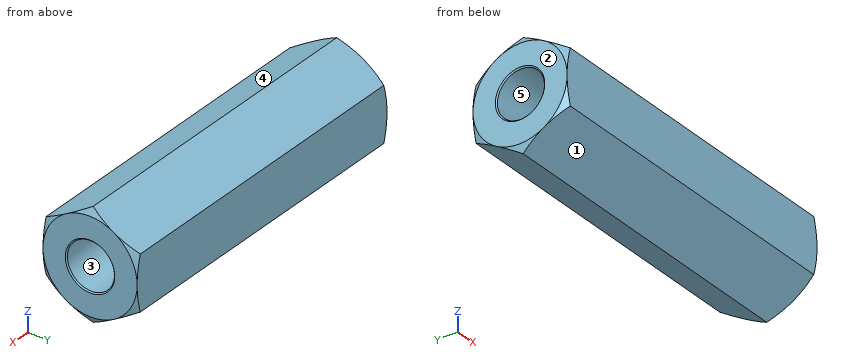
from build123d import *

# Parameters (mm, degrees)
BOSS_EXTRUDE1_DEPTH = 28
SKETCH4_OUTSIDE_W   = 117.808
SKETCH4_OUTSIDE_H   = 116.57
SKETCH4_OUTSIDE_R   = 4
CUT_EXTRUDE1_DEPTH  = 29
CUT_EXTRUDE1_TAPER  = 60
SKETCH5_OUTSIDE_W   = 117.808
SKETCH5_OUTSIDE_H   = 116.57
SKETCH5_OUTSIDE_R   = 4
CUT_EXTRUDE2_DEPTH  = 29
CUT_EXTRUDE2_TAPER  = 60


with BuildPart() as part:
    # Sketch2 → Boss-Extrude1 (new body)
    with BuildSketch(Plane(origin=(0, 0, 0), x_dir=(0, 0, -1), z_dir=(1, 0, 0))):
        Polygon((2.309401077, 4), (-2.309401077, 4), (-4.618802154, 0), (-2.309401077, -4), (2.309401077, -4), (4.618802154, 0), align=None)
    extrude(amount=BOSS_EXTRUDE1_DEPTH)

    # Sketch3 → Cut-Revolve1 (revolve, cut)
    with BuildSketch(Plane.XY):
        Polygon((0, 2.1), (0.1, 2), (11.1, 2), (11.1, 0), (0, 0), align=None)
        Polygon((28, 0), (16.9, 0), (16.9, 2), (27.9, 2), (28, 2.1), align=None)
    revolve(axis=Axis((0, 0, 0), (1, 0, 0)), mode=Mode.SUBTRACT)

    # Sketch4 outside → Cut-Extrude1 (cut, through all)
    with BuildSketch(Plane.ZY):
        Rectangle(SKETCH4_OUTSIDE_W, SKETCH4_OUTSIDE_H)
        Circle(SKETCH4_OUTSIDE_R, mode=Mode.SUBTRACT)
    extrude(amount=-CUT_EXTRUDE1_DEPTH, taper=CUT_EXTRUDE1_TAPER, mode=Mode.SUBTRACT)

    # Sketch5 outside → Cut-Extrude2 (cut, through all)
    with BuildSketch(Plane(origin=(28, 0, 0), x_dir=(0, 0, -1), z_dir=(1, 0, 0))):
        Rectangle(SKETCH5_OUTSIDE_W, SKETCH5_OUTSIDE_H)
        Circle(SKETCH5_OUTSIDE_R, mode=Mode.SUBTRACT)
    extrude(amount=-CUT_EXTRUDE2_DEPTH, taper=CUT_EXTRUDE2_TAPER, mode=Mode.SUBTRACT)


solid = part.part
CAD build for the part. Positions are in the model's coordinates, mm. Face numbers are marked on the shaded views. A direction names the side the tool comes from. Coordinates: 2 decimals unless noted, no trailing zeros. Loops run counter-clockwise (first coordinate to the right, second up) from the corner with the lowest first, then second, coordinate; pieces in that order, holes last. Notation, with made-up numbers: (0.25, -12) - (12.25, -12) arc R24 ccw to (12.25, 2) - close; hole circle Ø9 at (2.5, -40). An arc over 180 degrees is marked (long way). Write item = value, one per line. Start each with the question number.
Q1. Pull direction Z, two halves, no side cores. Call the marked faces 1, 2 and 3: pulls with the +Z half, pulls with the -Z half, needs draft (parallel to the pull), parting line crosses it, or undercut.
Q2. Cut at A-A, the plane x = 9.75. List the corners of the cut face in (y, z).
Q3. Flat gauge pins, fed straight in: pin 1 Ø3 at (y, z) = (0, 0) entering from +X; pin 2 Ø1 at (x, y) = (23.5, -2) entering from +Z; pin 3 Ø2 at (x, y) = (7.5, -1.5) entering from +Z. Where does each tip first touch, or does it go through?
Q4. Drill centre lines: L1, parallel to X at y = -1, z = -1; L2, parallel to Z at x = 5.25, y = 0.75; L3, parallel to Y at x = 9.5, z = -1. Where is each one in solid material? Low to high.
Q5. Which spindle directions (+Z, -Z, +X, -X, +Y, -Y) get a long thin tool onto all of the face, cutting with end or side? Do the marked faces 4 and 5. Say none if no direction does.
Computed:
q1.face_1 = pulls with the -Z half
q1.face_2 = needs draft
q1.face_3 = undercut
q2.outline = (-4, -2.31) - (0, -4.62) - (4, -2.31) - (4, 2.31) - (0, 4.62) - (-4, 2.31) - close; hole circle Ø4 at (0, 0)
q3.pin_1 = 16.9
q3.pin_2 = 3.75
q3.pin_3 = 4.33
q4.L1 = 11.1 to 16.9
q4.L2 = -4.19 to -1.85, 1.85 to 4.19
q4.L3 = -4 to -1.73, 1.73 to 4
q5.face_4 = +Z, +X, -X, -Y
q5.face_5 = -X
